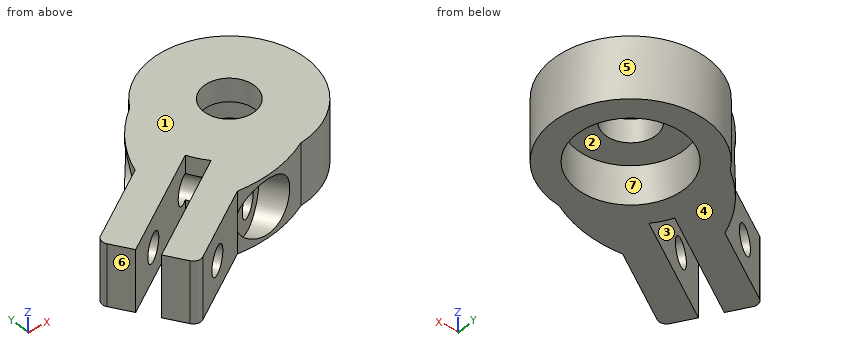
```python
from build123d import *

# Parameters (mm, degrees)
SKETCH1_R               = 10
SKETCH1_R_2             = 6.925
BOSS_EXTRUDE1_DEPTH     = 5
BOSS_EXTRUDE2_START     = 3
SKETCH3_R               = 10
SKETCH3_R_2             = 3.272939667
BOSS_EXTRUDE2_DEPTH     = 3
BOSS_EXTRUDE3_START     = -8
BOSS_EXTRUDE3_DEPTH     = 8
CUT_EXTRUDE1_DEPTH      = 32.194168296
CUT_EXTRUDE1_DEPTH_BACK = 32.194168296
SKETCH5_R               = 1.75
SKETCH6_R               = 3.5
CUT_EXTRUDE2_DEPTH      = 32.194168296


with BuildPart() as part:
    # Sketch1 → Boss-Extrude1 (new body)
    with BuildSketch(Plane.XY):
        Circle(SKETCH1_R)
        Circle(SKETCH1_R_2, mode=Mode.SUBTRACT)
    extrude(amount=-BOSS_EXTRUDE1_DEPTH)

    # Sketch3 → Boss-Extrude2 (add)
    with BuildSketch(Plane.XY.offset(BOSS_EXTRUDE2_START)):
        Circle(SKETCH3_R)
        Circle(SKETCH3_R_2, mode=Mode.SUBTRACT)
    extrude(amount=-BOSS_EXTRUDE2_DEPTH)

    # Sketch4 → Boss-Extrude3 (add)
    with BuildSketch(Plane(origin=(0, 0, -5), x_dir=(-1, 0, 0), z_dir=(0, 0, -1)).offset(BOSS_EXTRUDE3_START)):
        with BuildLine():
            add(Edge.make_bspline(
                [(8.498319818, 5.270537), (12.759977843, 2.15344034), (14.492799423, -2.673176889)],
                knots=[0, 0, 0, 1, 1, 1], degree=2))
            ThreePointArc((8.498319818, 5.270537), (9.617255278, 2.740146147), (10, 0))
            ThreePointArc((10, 0), (9.78187229, -2.077251673), (9.137005098, -4.063882115))
            Line((9.137005098, -4.063882115), (22.594413904, -12.387282242))
            Line((22.594413904, -12.387282242), (24.172466522, -9.835861082))
            ThreePointArc((24.172466522, -9.835861082), (24.295319106, -9.080418377), (23.848010342, -8.459369823))
            Line((23.848010342, -8.459369823), (14.492799423, -2.673176889))
        make_face()
        with BuildLine():
            add(Edge.make_bspline(
                [(-0.920254083, -9.957566591), (3.772003923, -12.378462192), (8.864411751, -11.773245691)],
                knots=[0, 0, 0, 1, 1, 1], degree=2))
            Line((8.864411751, -11.773245691), (18.219622669, -17.559438625))
            ThreePointArc((18.219622669, -17.559438625), (18.975065374, -17.682291209), (19.596113929, -17.234982445))
            Line((19.596113929, -17.234982445), (21.174166547, -14.683561285))
            Line((21.174166547, -14.683561285), (7.716757741, -6.360161159))
            ThreePointArc((7.716757741, -6.360161159), (3.844924831, -9.231281224), (-0.920254083, -9.957566591))
        make_face()
    extrude(amount=BOSS_EXTRUDE3_DEPTH)

    # Sketch5 → Cut-Extrude1 (cut, two sides: drawn at the far end of the back side and taken through both)
    with BuildSketch(Plane(origin=(2.814193836, -4.550034401, 0), x_dir=(0.8504737198659906, 0.526017539457863, 0), z_dir=(0.526017539457863, -0.8504737198659906, 0)).offset(-CUT_EXTRUDE1_DEPTH_BACK)):
        with Locations((-10.421994874, -1)):
            Circle(SKETCH5_R)
        with Locations((-20.108842695, -1)):
            Circle(SKETCH5_R)
    extrude(amount=CUT_EXTRUDE1_DEPTH + CUT_EXTRUDE1_DEPTH_BACK, mode=Mode.SUBTRACT)

    # Sketch6 → Cut-Extrude2 (cut, through all)
    with BuildSketch(Plane(origin=(2.814193836, -4.550034401, 0), x_dir=(0.8504737198659906, 0.526017539457863, 0), z_dir=(0.526017539457863, -0.8504737198659906, 0))):
        with Locations((-10.421994874, -1)):
            Circle(SKETCH6_R)
    cut_extrude2 = extrude(amount=CUT_EXTRUDE2_DEPTH, mode=Mode.SUBTRACT)

    # Mirror1: Cut-Extrude2 across plane
    add(cut_extrude2.mirror(Plane(origin=(0, 0, 0), x_dir=(0, 0, 1), z_dir=(0.526017539457863, -0.8504737198659906, 0))), mode=Mode.SUBTRACT)


solid = part.part
```
The model under review builds one solid part; all positions refer to its coordinate system, in mm. Face numbers are marked on the shaded views. A direction names the side the tool comes from. Give positions to 0.01 mm unless a question says otherwise; leave off trailing zeros. Write each loop counter-clockwise with the first axis right and the second up, starting at its lowest first coordinate (ties: lowest second). Pieces come first, ordered by that corner, then holes.
(1) Consider section A-A, the plane y = 6.5. Give the boundary of the cut face in (x, z), and give its area (3 significant figures).
(2) To check wall thickness, follow L1, parallel to X at y = -6, z = -2.25; L2, parallel to X at y = -4.5, z = -0.75; L3, parallel to X at y = 5, z = -3.5. State the ranges of each line that lie inside material, in increasing order.
(3) Tool access review of the marked faces 1, 2 and 3: name each direction out of +Z, -Z, +X, -X, +Y, -Y from which nothing blocks a thin tool from reaching the whole face with its end or side.
(4) The part is to be moulded in two halves that separate along X. For the marked faces 4, 5, 6 and 7, say which applies: released by +X, released by -X, zero draft, split by the parting line, or undercut.
(5) For P1, Ø5, axis at x = -3.5, y = 2, coming from the -Z side; P2, Ø3, axis at y = -0.5, z = 0, coming from the -X side; P3, Ø2, axis at x = -17.5, z = 1.5, coming from the +Y side; P4, Ø11, axis at x = 1, y = -3, coming from the -Z side, all flat-tipped, find the tip position at first contact; note any pin that passes through.
Returned:
1. outline: (-7.6, -5) - (-2.39, -5) - (-2.39, 0) - (2.39, 0) - (2.39, -5) - (7.6, -5) - (7.6, 3) - (-7.6, 3) - close
1. area: 97.7 mm2
2. L1: x = -18.49 to -12.27, -7.1 to -3.46, 3.46 to 8
2. L2: x = -17.45 to -11.51, -7.43 to -5.26, 5.26 to 8.93
2. L3: x = -8.86 to -4.79, 4.79 to 8.66
3. face 1: +Z, +X, -X, +Y, -Y
3. face 2: -Z
3. face 3: +Z, -Z
4. face 4: zero draft
4. face 5: split by the parting line
4. face 6: released by -X
4. face 7: undercut
5. P1: stops at z = 0
5. P2: stops at x = -13.4
5. P3: stops at y = -3.91
5. P4: stops at z = -5
